Can you work these out from the model? Positions are in its coordinate system, mm. Face numbers are marked on the shaded views. A direction names the side the tool comes from. Give positions to 0.01 mm unless a question says otherwise; leave off trailing zeros. Order: outer loops, then holes, each group sorted by start corner. A loop starts at its lowest first (then second) coordinate and runs counter-clockwise, first axis right, second up. Notation, with made-up numbers: (-34, -26.5) -> (-18, -26.5) arc R22 ccw to (-18, -13.5) -> close; hole circle Ø10 at (48, 27.25). An arc over 180 degrees is marked (long way). Answer as a JSON object with one key per item and string values.
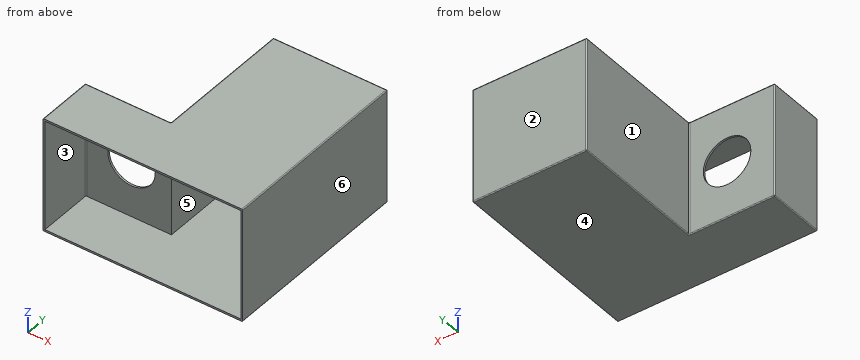
```python
from build123d import *

# Parameters (mm, degrees)
SKETCH1_W           = 210
SKETCH1_H           = 205
BOSS_EXTRUDE1_DEPTH = 120
SKETCH2_W           = 90
SKETCH2_H           = 145
CUT_EXTRUDE1_DEPTH  = 120
SKETCH3_W           = 88
SKETCH3_H           = 116
CUT_EXTRUDE4_DEPTH  = 58
SKETCH6_W           = 116
SKETCH6_H           = 116
CUT_EXTRUDE6_DEPTH  = 203
SKETCH7_W           = 2
SKETCH7_H           = 116
CUT_EXTRUDE7_DEPTH  = 58
FILLET1_R           = 1
FILLET2_R           = 1
FILLET3_R           = 1
SKETCH8_R           = 25
CUT_EXTRUDE8_DEPTH  = 58


with BuildPart() as part:
    # Sketch1 → Boss-Extrude1 (new body)
    with BuildSketch(Plane.XY):
        Rectangle(SKETCH1_W, SKETCH1_H)
    extrude(amount=BOSS_EXTRUDE1_DEPTH)

    # Sketch2 → Cut-Extrude1 (cut)
    with BuildSketch(Plane.XY.offset(120)):
        with Locations((-60, 30)):
            Rectangle(SKETCH2_W, SKETCH2_H)
    extrude(amount=-CUT_EXTRUDE1_DEPTH, mode=Mode.SUBTRACT)

    # Sketch3 → Cut-Extrude4 (cut)
    with BuildSketch(Plane.XZ.offset(102.5)):
        with Locations((-59, 60)):
            Rectangle(SKETCH3_W, SKETCH3_H)
    extrude(amount=-CUT_EXTRUDE4_DEPTH, mode=Mode.SUBTRACT)

    # Sketch6 → Cut-Extrude6 (cut)
    with BuildSketch(Plane(origin=(0, -102.5, 0), x_dir=(-1, 0, 0), z_dir=(0, -1, 0))):
        with Locations((-45, -60)):
            Rectangle(SKETCH6_W, SKETCH6_H)
    extrude(amount=-CUT_EXTRUDE6_DEPTH, mode=Mode.SUBTRACT)

    # Sketch7 → Cut-Extrude7 (cut)
    with BuildSketch(Plane(origin=(0, -102.5, 0), x_dir=(-1, 0, 0), z_dir=(0, -1, 0))):
        with Locations((14, -60)):
            Rectangle(SKETCH7_W, SKETCH7_H)
    extrude(amount=-CUT_EXTRUDE7_DEPTH, mode=Mode.SUBTRACT)

    # Fillet1
    fillet1_edges = [part.edges().sort_by_distance(p)[0] for p in [
        (-105, -72.5, 0),
        (-105, -72.5, 120),
        (-15, 30, 0),
        (-15, 102.5, 60),
        (-60, -42.5, 0),
        (-15, -42.5, 60),
        (-60, -42.5, 120),
        (-15, 30, 120),
        (-103, -44.5, 60),
        (105, 0, 120),
        (45, 102.5, 120),
    ]]
    fillet(fillet1_edges, radius=FILLET1_R)

    # Fillet2
    # the kernel refuses this fillet: 1 mm, written as the material it takes off along each edge
    with BuildSketch(Plane(origin=(-14, 101.5, 1), x_dir=(0, 1, 0), z_dir=(0, 0, -1))) as fillet2_piece_1_section:
        Polygon((0, 0), (FILLET2_R, 0), (FILLET2_R, -FILLET2_R), (0, -FILLET2_R), align=None)
    fillet2_piece_1 = extrude(amount=FILLET2_R, mode=Mode.PRIVATE)
    fillet2_piece_1 = fillet2_piece_1 - Plane(origin=(-14, 101.5, 1), x_dir=(0.7071067811865476, -0.7071067811865475, 0), z_dir=(0, 0, -1)) * Sphere(FILLET2_R, mode=Mode.PRIVATE)
    add(fillet2_piece_1, mode=Mode.SUBTRACT)
    with BuildSketch(Plane(origin=(104, 101.5, 119), x_dir=(0, 1, 0), z_dir=(1, 0, 0))) as fillet2_piece_2_section:
        Polygon((0, 0), (FILLET2_R, 0), (FILLET2_R, FILLET2_R), (0, FILLET2_R), align=None)
    fillet2_piece_2 = extrude(amount=FILLET2_R, mode=Mode.PRIVATE)
    fillet2_piece_2 = fillet2_piece_2 - Plane(origin=(104, 101.5, 119), x_dir=(0, -0.7071067811865475, -0.7071067811865475), z_dir=(1, 0, 0)) * Sphere(FILLET2_R, mode=Mode.PRIVATE)
    add(fillet2_piece_2, mode=Mode.SUBTRACT)
    with BuildSketch(Plane(origin=(104, 101.5, 1), x_dir=(1, 0, 0), z_dir=(0, 0, -1))) as fillet2_piece_3_section:
        Polygon((0, 0), (FILLET2_R, 0), (FILLET2_R, -FILLET2_R), (0, -FILLET2_R), align=None)
    fillet2_piece_3 = extrude(amount=FILLET2_R, mode=Mode.PRIVATE)
    fillet2_piece_3 = fillet2_piece_3 - Plane(origin=(104, 101.5, 1), x_dir=(-0.7071067811865475, -0.7071067811865475, 0), z_dir=(0, 0, -1)) * Sphere(FILLET2_R, mode=Mode.PRIVATE)
    add(fillet2_piece_3, mode=Mode.SUBTRACT)
    with BuildSketch(Plane(origin=(104, 102.5, 0), x_dir=(0, -1, 0), z_dir=(-1, 0, 0))) as fillet2_piece_4:
        with BuildLine():
            CenterArc((FILLET2_R, FILLET2_R), FILLET2_R, 180, 90)
            Line((0, FILLET2_R), (0, 0))
            Line((0, 0), (FILLET2_R, 0))
        make_face()
    extrude(amount=118, mode=Mode.SUBTRACT)
    with BuildSketch(Plane(origin=(105, -105, 0), x_dir=(-1, 0, 0), z_dir=(0, 1, 0))) as fillet2_piece_5:
        with BuildLine():
            CenterArc((FILLET2_R, FILLET2_R), FILLET2_R, 180, 90)
            Line((0, FILLET2_R), (0, 0))
            Line((0, 0), (FILLET2_R, 0))
        make_face()
    extrude(amount=206.5, mode=Mode.SUBTRACT)
    with BuildSketch(Plane(origin=(105, 102.5, 1), x_dir=(0, -1, 0), z_dir=(0, 0, 1))) as fillet2_piece_6:
        with BuildLine():
            CenterArc((FILLET2_R, -FILLET2_R), FILLET2_R, 90, 90)
            Line((0, -FILLET2_R), (0, 0))
            Line((0, 0), (FILLET2_R, 0))
        make_face()
    extrude(amount=118, mode=Mode.SUBTRACT)

    # Fillet3
    # the kernel refuses this fillet: 1 mm, written as the material it takes off along each edge
    with BuildSketch(Plane(origin=(-104, -43.5, 1), x_dir=(0, 1, 0), z_dir=(-1, 0, 0))) as fillet3_piece_1_section:
        Polygon((0, 0), (FILLET3_R, 0), (FILLET3_R, FILLET3_R), (0, FILLET3_R), align=None)
    fillet3_piece_1 = extrude(amount=FILLET3_R, mode=Mode.PRIVATE)
    fillet3_piece_1 = fillet3_piece_1 - Plane(origin=(-104, -43.5, 1), x_dir=(0, -0.7071067811865475, 0.7071067811865475), z_dir=(-1, 0, 0)) * Sphere(FILLET3_R, mode=Mode.PRIVATE)
    add(fillet3_piece_1, mode=Mode.SUBTRACT)
    with BuildSketch(Plane(origin=(-104, -43.5, 119), x_dir=(0, 1, 0), z_dir=(-1, 0, 0))) as fillet3_piece_2_section:
        Polygon((0, 0), (FILLET3_R, 0), (FILLET3_R, -FILLET3_R), (0, -FILLET3_R), align=None)
    fillet3_piece_2 = extrude(amount=FILLET3_R, mode=Mode.PRIVATE)
    fillet3_piece_2 = fillet3_piece_2 - Plane(origin=(-104, -43.5, 119), x_dir=(0, -0.7071067811865475, -0.7071067811865475), z_dir=(-1, 0, 0)) * Sphere(FILLET3_R, mode=Mode.PRIVATE)
    add(fillet3_piece_2, mode=Mode.SUBTRACT)
    with BuildSketch(Plane(origin=(-105, -42.5, 119), x_dir=(0, -1, 0), z_dir=(0, 0, -1))) as fillet3_piece_3:
        with BuildLine():
            CenterArc((FILLET3_R, -FILLET3_R), FILLET3_R, 90, 90)
            Line((0, -FILLET3_R), (0, 0))
            Line((0, 0), (FILLET3_R, 0))
        make_face()
    extrude(amount=118, mode=Mode.SUBTRACT)

    # Sketch8 → Cut-Extrude8 (cut)
    with BuildSketch(Plane(origin=(0, -42.5, 0), x_dir=(1, 0, 0), z_dir=(0, 1, 0))):
        with Locations(Location((-55, -60, 0), (0, 0, 270))):
            Circle(SKETCH8_R)
    extrude(amount=-CUT_EXTRUDE8_DEPTH, mode=Mode.SUBTRACT)


solid = part.part
```
1. Please list where these lines run through material, in increasing order: L1, parallel to X at y = -43.5, z = 60; L2, parallel to X at y = -43, z = 60; L3, parallel to X at y = -33.5, z = 16.
Worked answers:
{"L1": "-105 to -80, -30 to -13, 103 to 105", "L2": "-104.87 to -80, -30 to -13, 103 to 105", "L3": "-15 to -13, 103 to 105"}
2. If we section it at B-B on x = -55: Please give me the cut outline in (y, z), then the cut area to 3 significant figures.
Worked answers:
{"outline": "(-102.5, 0) -> (-43.5, 0) arc R1 ccw to (-42.5, 1) -> (-42.5, 35) -> (-44.5, 35) -> (-44.5, 2) -> (-102.5, 2) -> close; (-102.5, 118) -> (-44.5, 118) -> (-44.5, 85) -> (-42.5, 85) -> (-42.5, 119) arc R1 ccw to (-43.5, 120) -> (-102.5, 120) -> close", "area": "372 mm²"}
3. If we mould it in two halves opening along Z, with no side actions, what happens to the marked faces 4, 5 and 6? For each: +Z half, -Z half, draft (parallel to the pull), parting line (faces both ways), or undercut.
Worked answers:
{"face 4": "-Z half", "face 5": "undercut", "face 6": "draft"}
4. If we section it at C-C on y = -60: Please give me the cut outline in (x, z).
Worked answers:
{"outline": "(-105, 1) arc R1 ccw to (-104, 0) -> (104, 0) arc R1 ccw to (105, 1) -> (105, 119) arc R1 ccw to (104, 120) -> (-104, 120) arc R1 ccw to (-105, 119) -> close; hole (-103, 2) -> (103, 2) -> (103, 118) -> (-103, 118) -> close"}
5. Will these pins go through, and if not, where does the flat tip stop? pin 1 Ø6 at (y, z) = (37.5, 45) entering from -X; pin 2 Ø3 at (x, z) = (-66.5, 89.5) entering from +Y; pin 3 Ø1 at (x, z) = (-39, 87) entering from -Y.
Worked answers:
{"pin 1": "x = -15", "pin 2": "y = -42.5", "pin 3": "y = -44.5"}
6. For the marked faces 1, 2 and 3, which set-ups out of +Z, -Z, +X, -X, +Y, -Y let a thin tool reach every point of the face, with its end or its side?
Worked answers:
{"face 1": "+Z, -Z, -X, +Y", "face 2": "+Z, -Z, +X, -X, +Y", "face 3": "-Y"}
7. If we section it at D-D on z = 100.5: Please give me the cut outline in (x, y).
Worked answers:
{"outline": "(-105, -102.5) -> (-103, -102.5) -> (-103, -45.5) arc R1 cw to (-102, -44.5) -> (-13, -44.5) -> (-13, 100.5) -> (103, 100.5) -> (103, -102.5) -> (105, -102.5) -> (105, 101.5) arc R1 ccw to (104, 102.5) -> (-14, 102.5) arc R1 ccw to (-15, 101.5) -> (-15, -41.5) arc R1 cw to (-16, -42.5) -> (-104, -42.5) arc R1 ccw to (-105, -43.5) -> close"}
8. If we section it at A-A on z = 60: Please give me the cut outline in (x, y).
Worked answers:
{"outline": "(-105, -102.5) -> (-103, -102.5) -> (-103, -45.5) arc R1 cw to (-102, -44.5) -> (-80, -44.5) -> (-80, -42.5) -> (-104, -42.5) arc R1 ccw to (-105, -43.5) -> close; (-30, -44.5) -> (-13, -44.5) -> (-13, 100.5) -> (103, 100.5) -> (103, -102.5) -> (105, -102.5) -> (105, 101.5) arc R1 ccw to (104, 102.5) -> (-14, 102.5) arc R1 ccw to (-15, 101.5) -> (-15, -41.5) arc R1 cw to (-16, -42.5) -> (-30, -42.5) -> close"}
